Could you check a few things on this model? Use its own coordinates, in mm. Round coordinates to 2 decimals unless told otherwise and drop trailing zeros. Write each loop counter-clockwise with the first axis right and the second up, starting at its lowest first coordinate (ties: lowest second). Pieces come first, ordered by that corner, then holes. Notation, with made-up numbers: M 21,84 L 33,84 A20 ccw 33,121 Z; hole C -15,-4 d2. An arc over 180 degrees is marked long. One line per item, written item: value. Start each with the question number.
(1) Thinking about a two-plate mould opening in Z: for faces 1 (the face through (92, 203, 0)), 2 (the face through (92, 203, 6.6)), which applies, released by +Z, released by -Z, zero draft, split by the parting line, or undercut?
(2) I want a section at A-A on y = 226. Please give me the cut outline in (x, z), and give its area (3 significant figures).
(3) If I drill on L1, parallel to X at y = 138, z = 2.25; L2, parallel to Y at x = 14, z = 3.5; L3, parallel to Y at x = 186, z = 0.5, over which ranges is the centre line in solid material (lowest first)?
(4) I'm going to push flat-ended pins straight in: pin 1 Ø1.3 at (y, z) = (262, 5) entering from +X; pin 2 Ø1.2 at (x, z) = (-1, 5) entering from +Y; pin 3 Ø1.7 at (y, z) = (262, 3.5) entering from -X. Where does each tip first touch, or does it pass through?
```python
from build123d import *

# Parameters (mm, degrees)
BOSS_EXTRUDE1_DEPTH = 6.6


with BuildPart() as part:
    # Model → Boss-Extrude1 (new body)
    with BuildSketch(Plane.XY):
        with BuildLine():
            Line((-6.5, 76), (-6.5, 66))
            ThreePointArc((-6.5, 66), (-5.767766953, 64.232233047), (-4, 63.5))
            Line((-4, 63.5), (0, 63.5))
            Line((0, 63.5), (0, 2))
            ThreePointArc((0, 2), (0.585786438, 0.585786438), (2, 0))
            Line((2, 0), (185.8, 0))
            ThreePointArc((185.8, 0), (187.214213562, 0.585786438), (187.8, 2))
            Line((187.8, 2), (187.8, 63.5))
            Line((187.8, 63.5), (191.8, 63.5))
            ThreePointArc((191.8, 63.5), (193.567766953, 64.232233047), (194.3, 66))
            Line((194.3, 66), (194.3, 76))
            ThreePointArc((194.3, 76), (193.567766953, 77.767766953), (191.8, 78.5))
            Line((191.8, 78.5), (187.8, 78.5))
            Line((187.8, 78.5), (187.8, 133.7375))
            Line((187.8, 133.7375), (176.8, 133.7375))
            Line((176.8, 133.7375), (176.8, 132.1525))
            ThreePointArc((176.8, 132.1525), (176.653553391, 131.798946609), (176.3, 131.6525))
            Line((176.3, 131.6525), (172.3, 131.6525))
            ThreePointArc((172.3, 131.6525), (171.946446609, 131.798946609), (171.8, 132.1525))
            Line((171.8, 132.1525), (171.8, 133.7375))
            Line((171.8, 133.7375), (167.3, 133.7375))
            ThreePointArc((167.3, 133.7375), (166.946446609, 133.883946609), (166.8, 134.2375))
            Line((166.8, 134.2375), (166.8, 136.7875))
            ThreePointArc((166.8, 136.7875), (166.946446609, 137.141053391), (167.3, 137.2875))
            Line((167.3, 137.2875), (171.8, 137.2875))
            Line((171.8, 137.2875), (171.8, 138.8725))
            ThreePointArc((171.8, 138.8725), (171.946446609, 139.226053391), (172.3, 139.3725))
            Line((172.3, 139.3725), (176.3, 139.3725))
            ThreePointArc((176.3, 139.3725), (176.653553391, 139.226053391), (176.8, 138.8725))
            Line((176.8, 138.8725), (176.8, 137.2875))
            Line((176.8, 137.2875), (187.8, 137.2875))
            Line((187.8, 137.2875), (187.8, 192.525))
            Line((187.8, 192.525), (191.8, 192.525))
            ThreePointArc((191.8, 192.525), (193.567766953, 193.257233047), (194.3, 195.025))
            Line((194.3, 195.025), (194.3, 205.025))
            ThreePointArc((194.3, 205.025), (193.567766953, 206.792766953), (191.8, 207.525))
            Line((191.8, 207.525), (187.8, 207.525))
            Line((187.8, 207.525), (187.8, 262.7625))
            Line((187.8, 262.7625), (176.8, 262.7625))
            Line((176.8, 262.7625), (176.8, 261.1775))
            ThreePointArc((176.8, 261.1775), (176.653553391, 260.823946609), (176.3, 260.6775))
            Line((176.3, 260.6775), (172.3, 260.6775))
            ThreePointArc((172.3, 260.6775), (171.946446609, 260.823946609), (171.8, 261.1775))
            Line((171.8, 261.1775), (171.8, 262.7625))
            Line((171.8, 262.7625), (167.3, 262.7625))
            ThreePointArc((167.3, 262.7625), (166.946446609, 262.908946609), (166.8, 263.2625))
            Line((166.8, 263.2625), (166.8, 265.8125))
            ThreePointArc((166.8, 265.8125), (166.946446609, 266.166053391), (167.3, 266.3125))
            Line((167.3, 266.3125), (171.8, 266.3125))
            Line((171.8, 266.3125), (171.8, 267.8975))
            ThreePointArc((171.8, 267.8975), (171.946446609, 268.251053391), (172.3, 268.3975))
            Line((172.3, 268.3975), (176.3, 268.3975))
            ThreePointArc((176.3, 268.3975), (176.653553391, 268.251053391), (176.8, 267.8975))
            Line((176.8, 267.8975), (176.8, 266.3125))
            Line((176.8, 266.3125), (187.8, 266.3125))
            Line((187.8, 266.3125), (187.8, 321.55))
            Line((187.8, 321.55), (191.8, 321.55))
            ThreePointArc((191.8, 321.55), (193.567766953, 322.282233047), (194.3, 324.05))
            Line((194.3, 324.05), (194.3, 334.05))
            ThreePointArc((194.3, 334.05), (193.567766953, 335.817766953), (191.8, 336.55))
            Line((191.8, 336.55), (187.8, 336.55))
            Line((187.8, 336.55), (187.8, 398.05))
            ThreePointArc((187.8, 398.05), (187.214213562, 399.464213562), (185.8, 400.05))
            Line((185.8, 400.05), (2, 400.05))
            ThreePointArc((2, 400.05), (0.585786438, 399.464213562), (0, 398.05))
            Line((0, 398.05), (0, 336.55))
            Line((0, 336.55), (-4, 336.55))
            ThreePointArc((-4, 336.55), (-5.767766953, 335.817766953), (-6.5, 334.05))
            Line((-6.5, 334.05), (-6.5, 324.05))
            ThreePointArc((-6.5, 324.05), (-5.767766953, 322.282233047), (-4, 321.55))
            Line((-4, 321.55), (0, 321.55))
            Line((0, 321.55), (0, 266.3125))
            Line((0, 266.3125), (11, 266.3125))
            Line((11, 266.3125), (11, 267.8975))
            ThreePointArc((11, 267.8975), (11.146446609, 268.251053391), (11.5, 268.3975))
            Line((11.5, 268.3975), (15.5, 268.3975))
            ThreePointArc((15.5, 268.3975), (15.853553391, 268.251053391), (16, 267.8975))
            Line((16, 267.8975), (16, 266.3125))
            Line((16, 266.3125), (20.5, 266.3125))
            ThreePointArc((20.5, 266.3125), (20.853553391, 266.166053391), (21, 265.8125))
            Line((21, 265.8125), (21, 263.2625))
            ThreePointArc((21, 263.2625), (20.853553391, 262.908946609), (20.5, 262.7625))
            Line((20.5, 262.7625), (16, 262.7625))
            Line((16, 262.7625), (16, 261.1775))
            ThreePointArc((16, 261.1775), (15.853553391, 260.823946609), (15.5, 260.6775))
            Line((15.5, 260.6775), (11.5, 260.6775))
            ThreePointArc((11.5, 260.6775), (11.146446609, 260.823946609), (11, 261.1775))
            Line((11, 261.1775), (11, 262.7625))
            Line((11, 262.7625), (0, 262.7625))
            Line((0, 262.7625), (0, 207.525))
            Line((0, 207.525), (-4, 207.525))
            ThreePointArc((-4, 207.525), (-5.767766953, 206.792766953), (-6.5, 205.025))
            Line((-6.5, 205.025), (-6.5, 195.025))
            ThreePointArc((-6.5, 195.025), (-5.767766953, 193.257233047), (-4, 192.525))
            Line((-4, 192.525), (0, 192.525))
            Line((0, 192.525), (0, 137.2875))
            Line((0, 137.2875), (11, 137.2875))
            Line((11, 137.2875), (11, 138.8725))
            ThreePointArc((11, 138.8725), (11.146446609, 139.226053391), (11.5, 139.3725))
            Line((11.5, 139.3725), (15.5, 139.3725))
            ThreePointArc((15.5, 139.3725), (15.853553391, 139.226053391), (16, 138.8725))
            Line((16, 138.8725), (16, 137.2875))
            Line((16, 137.2875), (20.5, 137.2875))
            ThreePointArc((20.5, 137.2875), (20.853553391, 137.141053391), (21, 136.7875))
            Line((21, 136.7875), (21, 134.2375))
            ThreePointArc((21, 134.2375), (20.853553391, 133.883946609), (20.5, 133.7375))
            Line((20.5, 133.7375), (16, 133.7375))
            Line((16, 133.7375), (16, 132.1525))
            ThreePointArc((16, 132.1525), (15.853553391, 131.798946609), (15.5, 131.6525))
            Line((15.5, 131.6525), (11.5, 131.6525))
            ThreePointArc((11.5, 131.6525), (11.146446609, 131.798946609), (11, 132.1525))
            Line((11, 132.1525), (11, 133.7375))
            Line((11, 133.7375), (0, 133.7375))
            Line((0, 133.7375), (0, 78.5))
            Line((0, 78.5), (-4, 78.5))
            ThreePointArc((-4, 78.5), (-5.767766953, 77.767766953), (-6.5, 76))
        make_face()
    extrude(amount=BOSS_EXTRUDE1_DEPTH)


solid = part.part
```
Found:
1. face 1: released by -Z
1. face 2: released by +Z
2. outline: M 0,0 L 187.8,0 L 187.8,6.6 L 0,6.6 Z
2. area: 1,240 mm²
3. L1: x = 0 to 11, 16 to 171.8, 176.8 to 187.8
3. L2: y = 0 to 131.65, 139.37 to 260.68, 268.4 to 400.05
3. L3: y = 0.01 to 133.74, 137.29 to 262.76, 266.31 to 400.04
4. pin 1: stops at x = 187.8
4. pin 2: stops at y = 336.55
4. pin 3: stops at x = 0
